Geometry check sheet. Reference: the model listing, model coordinates, mm. Face numbers are marked on the shaded views. Round coordinates to 2 decimals unless told otherwise and drop trailing zeros. Order: outer loops, then holes, each group sorted by start corner. A loop starts at its lowest first (then second) coordinate and runs counter-clockwise, first axis right, second up. Notation, with made-up numbers: (28.5, 56) - (59.5, 56) arc R21 ccw to (59.5, 62) - close; hole circle Ø8 at (22.5, -2.5). An arc over 180 degrees is marked (long way). Return JSON: item names as keys, results as strings. Group by question number.
Q1. Sectioned sample at D-D, the plane y = 24. Record the cut outline in (x, z).
Q2. Draft check along Z on the marked faces 1, 2 and 3. Enter one of: pulls with the +Z half, pulls with the -Z half, needs draft (parallel to the pull), parting line crosses it, or undercut.
Q3. Sectioned sample at A-A, the plane y = 11. Record the cut outline in (x, z).
Q4. Material ranges on line 1 along Y through (x, z) = (-12, 24); line 2 along Z through (x, y) = (21.5, 22); line 3 along X through (y, z) = (16.5, -6.5), recorded low to high.
Q5. Gauge pin test, flat end, axial feed: pin 1 Ø4 at (y, z) = (45, -19.5) entering from +X. Record the tip position at first contact, or that the pin passes through.
Q6. Sectioned sample at C-C, the plane z = 15.5. Record the cut outline in (x, y).
Q7. Sectioned sample at B-B, the plane x = -18. Record the cut outline in (y, z).
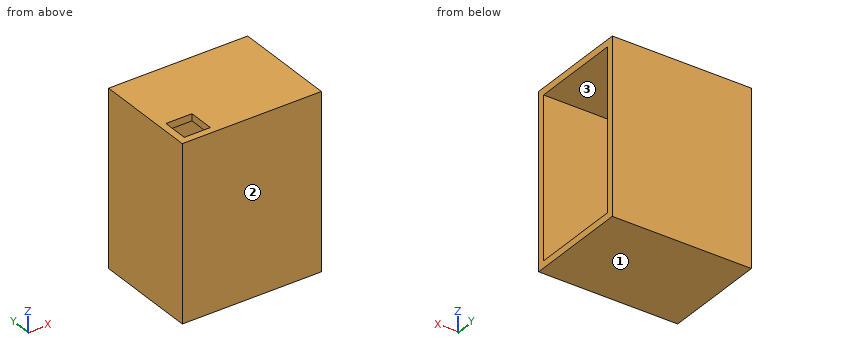
```python
from build123d import *

# Parameters (mm, degrees)
SKETCH1_W           = 80
SKETCH1_H           = 100
BOSS_EXTRUDE1_DEPTH = 60
SKETCH4_W           = 92
SKETCH4_H           = 52
CUT_EXTRUDE1_DEPTH  = 76
SKETCH5_W           = 15
SKETCH5_H           = 15
CUT_EXTRUDE2_DEPTH  = 4


with BuildPart() as part:
    # Sketch1 → Boss-Extrude1 (new body)
    with BuildSketch(Plane(origin=(0, 0, 0), x_dir=(1, 0, 0), z_dir=(0, 1, 0))):
        Rectangle(SKETCH1_W, SKETCH1_H)
    extrude(amount=BOSS_EXTRUDE1_DEPTH)

    # Sketch4 → Cut-Extrude1 (cut)
    with BuildSketch(Plane(origin=(40, 0, 0), x_dir=(0, 0, -1), z_dir=(1, 0, 0))):
        with Locations((0, 30)):
            Rectangle(SKETCH4_W, SKETCH4_H)
    extrude(amount=-CUT_EXTRUDE1_DEPTH, mode=Mode.SUBTRACT)

    # Sketch5 → Cut-Extrude2 (cut)
    with BuildSketch(Plane.XY.offset(50)):
        with Locations((-28.5, 11.5)):
            Rectangle(SKETCH5_W, SKETCH5_H)
    extrude(amount=-CUT_EXTRUDE2_DEPTH, mode=Mode.SUBTRACT)


solid = part.part
```
Reply:
{
 "1": {"outline": "(-40, -50) - (40, -50) - (40, -46) - (-36, -46) - (-36, 46) - (40, 46) - (40, 50) - (-40, 50) - close"},
 "2": {"face 1": "pulls with the -Z half", "face 2": "needs draft", "face 3": "undercut"},
 "3": {"outline": "(-40, -50) - (40, -50) - (40, -46) - (-36, -46) - (-36, 50) - (-40, 50) - close; (-21, 46) - (40, 46) - (40, 50) - (-21, 50) - close"},
 "4": {"line 1": "0 to 4, 56 to 60", "line 2": "-50 to -46, 46 to 50", "line 3": "-40 to -36"},
 "5": {"pin 1": "x = -36"},
 "6": {"outline": "(-40, 0) - (40, 0) - (40, 4) - (-36, 4) - (-36, 56) - (40, 56) - (40, 60) - (-40, 60) - close"},
 "7": {"outline": "(0, -50) - (60, -50) - (60, 50) - (0, 50) - close; hole (4, -46) - (56, -46) - (56, 46) - (4, 46) - close"}
}
